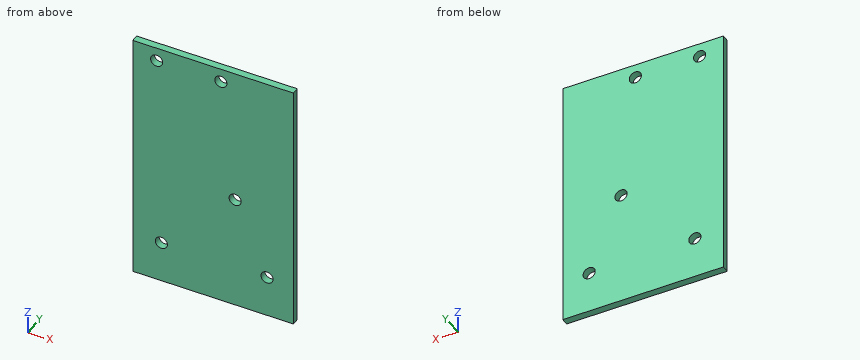
```python
from build123d import *

# Parameters (mm, degrees)
SKETCH1_W                = 45
SKETCH1_H                = 72
BASE_FLANGE1_DEPTH       = 2
NEED_TO_REPOSITION_D     = 3.4
NEED_TO_REPOSITION_DEPTH = 12
NEED_TO_REPOSITION_TIP   = 1.021463052


# Sheet-metal steps are written as plain solids
with BuildPart() as part:
    # Sketch1 → Base-Flange1 (new body)
    with BuildSketch(Plane(origin=(0, 0, 0), x_dir=(1, 0, 0), z_dir=(0, 1, 0))):
        Rectangle(SKETCH1_W, SKETCH1_H)
    extrude(amount=-BASE_FLANGE1_DEPTH)

    # Need to Reposition
    with Locations(Plane(origin=(0, -2, 0), x_dir=(-1, 0, 0), z_dir=(0, -1, 0))):
        with Locations((-2.172321578, -32.098), (15.827678422, -32.098), (-6.172321578, 3.23), (-15.109631715, 24.190770957), (14.504316145, 24.190770957)):
            Hole(NEED_TO_REPOSITION_D / 2, depth=NEED_TO_REPOSITION_DEPTH)
            with Locations((0, 0, -(NEED_TO_REPOSITION_DEPTH + NEED_TO_REPOSITION_TIP / 2))):  # 118° drill point
                Cone(0, NEED_TO_REPOSITION_D / 2, NEED_TO_REPOSITION_TIP, mode=Mode.SUBTRACT)


solid = part.part
```
Build history of the part. All positions in model axes, mm. Round coordinates to 2 decimals unless told otherwise and drop trailing zeros. Write each loop counter-clockwise with the first axis right and the second up, starting at its lowest first coordinate (ties: lowest second). Pieces come first, ordered by that corner, then holes. Notation, with made-up numbers: (78.5, -5) -> (131.5, -5) arc R16 cw to (131.5, 24) -> close; hole circle Ø10 at (56, -29.5). An arc over 180 degrees is marked (long way). Put each result on its own line as item: value.
Item 1: Slice it at A-A, the plane z = -3.23. Give the cut face in (x, y), plus the area to 3 significant figures.
Here are the results:
outline: (-22.5, -2) -> (4.47, -2) -> (4.47, 0) -> (-22.5, 0) -> close; (7.87, -2) -> (22.5, -2) -> (22.5, 0) -> (7.87, 0) -> close
area: 83.2 mm^2
Item 2: Flat gauge pins, fed straight in: P1, Ø2.5, axis at x = 6.17, z = -3.23, coming from the +Y side; P2, Ø4.5, axis at x = -15.83, z = 32.1, coming from the -Y side. Where does each tip first touch, or does it go through?
Here are the results:
P1: passes through
P2: stops at y = -2
Item 3: Slice it at B-B, the plane x = 1.5. Give the cut face in (y, z).
Here are the results:
outline: (-2, -36) -> (0, -36) -> (0, 30.54) -> (-2, 30.54) -> close; (-2, 33.66) -> (0, 33.66) -> (0, 36) -> (-2, 36) -> close
Item 4: Wall check: probe 1 along X at (y, z) = (-0.6, 33.5); probe 2 along Z at (x, y) = (16, -0.9); probe 3 along Z at (x, y) = (7, -1.5). Give the ranges that are in metal, low to high. Write a range as from..to.
Here are the results:
probe 1: x = -22.5..-16.79, -14.87..1.21, 3.13..22.5
probe 2: z = -36..-25.64, -22.74..36
probe 3: z = -36..-4.71, -1.75..36
